Verification items for the finished model (mm, model axes). A direction names the side the tool comes from. Round coordinates to 2 decimals unless told otherwise and drop trailing zeros. Write each loop counter-clockwise with the first axis right and the second up, starting at its lowest first coordinate (ties: lowest second). Pieces come first, ordered by that corner, then holes. Notation, with made-up numbers: (51, 49) - (110, 49) arc R15 cw to (110, 65) - close; hole circle Ø9 at (-19.5, -22). An arc over 180 degrees is marked (long way). Answer as a JSON object with one key per item and string values.
```python
from build123d import *

# Parameters (mm, degrees)
F0_R     = 50.8
F0_R_2   = 25.4
F1_DEPTH = 25.4
F2_W     = 150
F2_H     = 150
F2_R     = 50.8
F3_DEPTH = 25
F4_R     = 25.4
F4_R_2   = 22.5
F5_DEPTH = 25


# Not quite as in the source:
# - the program builds the solid bodies; features that only make, move or delete a surface that nothing else refers to are left out


with BuildPart() as f1:
    # F0 (on Top) → F1 (new body)
    with BuildSketch(Plane.XY):
        Circle(F0_R)
        Circle(F0_R_2, mode=Mode.SUBTRACT)
    extrude(amount=F1_DEPTH)

    # F2 (on Top) → F3 (join)
    with BuildSketch(Plane.XY):
        Rectangle(F2_W, F2_H)
        Circle(F2_R, mode=Mode.SUBTRACT)
    extrude(amount=F3_DEPTH)

    # F4 (on Top) → F5 (join)
    with BuildSketch(Plane.XY):
        Circle(F4_R)
        Circle(F4_R_2, mode=Mode.SUBTRACT)
    extrude(amount=F5_DEPTH)


solid = f1.part
```
1. Material ranges on probe 1 along Y at (x, z) = (0, 7.5); probe 2 along Y at (x, z) = (0, 25.1); probe 3 along Z at (x, y) = (27, -62.5), recorded low to high. Write a range as from..to.
Completed:
{"probe 1": "y = -75..-22.5, 22.5..75", "probe 2": "y = -50.8..-25.4, 25.4..50.8", "probe 3": "z = 0..25"}
2. Cross-section at D-D (y = -60). Record the boundary of the cut face in (x, z).
Completed:
{"outline": "(-75, 0) - (75, 0) - (75, 25) - (-75, 25) - close"}
3. Go/stop test with a flat-tipped pin: pin 1 (1.5 mm diameter, centred on x = -14.5, y = -16.5, fed in from +Z). Record where the tip stops, or that it passes through.
Completed:
{"pin 1": "stops at z = 25"}
4. Mould release check, pull along X, two halves, no side actions. Record for faces 1 (the face through (-75, -1, 12)), 2 (the face through (-1, 75, 12)), 3 (the face through (-15, -17, 25)), 4 (the face through (-11.012, -49.592, 25.197)): released by +X, released by -X, zero draft, split by the parting line, or undercut.
Completed:
{"face 1": "released by -X", "face 2": "zero draft", "face 3": "undercut", "face 4": "split by the parting line"}
5. Cross-section at A-A (y = 0). Record the boundary of the cut face in (x, z).
Completed:
{"outline": "(-75, 0) - (-22.5, 0) - (-22.5, 25) - (-25.4, 25) - (-25.4, 25.4) - (-50.8, 25.4) - (-50.8, 25) - (-75, 25) - close; (22.5, 0) - (75, 0) - (75, 25) - (50.8, 25) - (50.8, 25.4) - (25.4, 25.4) - (25.4, 25) - (22.5, 25) - close"}
6. Access from +Z, -Z, +X, -X, +Y, -Y to the whole of each face (thin tool, end or side, straight path). Record for faces 5 (the face through (-5.506, -24.796, 25.197)), 6 (the face through (-1, -75, 12)).
Completed:
{"face 5": "+Z", "face 6": "+Z, -Z, +X, -X, -Y"}
7. Cross-section at C-C (z = 16.25). Record the boundary of the cut face in (x, y).
Completed:
{"outline": "(-75, -75) - (75, -75) - (75, 75) - (-75, 75) - close; hole circle Ø45 at (0, 0)"}
